```python
from build123d import *

# Parameters (mm, degrees)
F1_DEPTH = 15


with BuildPart() as f1:
    # F0 (on Front) → F1 (new body)
    with BuildSketch(Plane.XZ):
        with BuildLine():
            Line((177, 0), (0, 0))
            Line((0, 0), (0, -1337))
            Line((0, -1337), (274, -1337))
            Line((274, -1337), (274, -1212))
            ThreePointArc((274, -1212), (322.5253137442, -1088.8902928279), (442, -1032))
            Line((442, -1032), (442, -1000))
            Line((442, -1000), (480, -967))
            Line((480, -967), (480, -937))
            Line((480, -937), (477, -887))
            add(Edge.make_bspline(
                [(477, -887), (477.3409901345, -865.6929372181), (477.0797844675, -851.0610734518), (476.1022594588, -737.3138139423), (476.5777735361, -793.1899508202), (474.0967013355, -723.7578035301), (464.8329395432, -637.3258006514), (461.2628948716, -536.660924146), (443.9915396348, -436.9186876346), (426.5757756979, -336.5383755873), (399.3587210867, -237.3522036261), (375.4775408132, -133.8744354339), (355.455463807, -69.1251180104), (340, -27)],
                knots=[0, 0, 0, 0, 0.0728496243, 0.1620736999, 0.2013801511, 0.2662309643, 0.3694203367, 0.4725712376, 0.576170853, 0.6801132511, 0.7847115324, 0.8893098137, 1, 1, 1, 1], degree=3))
            Line((340, -27), (177, 0))
        make_face()
        with BuildLine():
            ThreePointArc((85, -582), (86.4644660941, -578.4644660941), (90, -577))
            Line((90, -577), (360, -577))
            ThreePointArc((360, -577), (363.5355339059, -578.4644660941), (365, -582))
            Line((365, -582), (365, -732))
            ThreePointArc((365, -732), (363.5355339059, -735.5355339059), (360, -737))
            Line((360, -737), (90, -737))
            ThreePointArc((90, -737), (86.4644660941, -735.5355339059), (85, -732))
            Line((85, -732), (85, -582))
        make_face(mode=Mode.SUBTRACT)
    extrude(amount=F1_DEPTH)


solid = f1.part
```
For this review, take the finished solid that the model builds, in its own axes (mm). Round coordinates to 2 decimals unless told otherwise and drop trailing zeros. Order: outer loops, then holes, each group sorted by start corner. A loop starts at its lowest first (then second) coordinate and runs counter-clockwise, first axis right, second up. Notation, with made-up numbers: (12, 64.5) -> (16, 64.5) arc R23 cw to (16, 84.5) -> close; hole circle Ø9 at (3, -4.75). An arc over 180 degrees is marked (long way). Use a Markdown table: item, result.
Item 1: For line 1 along Z through (x, y) = (99, -4.5); line 2 along Z through (x, y) = (324, -14); line 3 along X through (y, z) = (-9, -1021), list the stretches that pass through material, from the lowest coordinate up. Write a range as [from, to].
Resolved:
| item | result |
|---|---|
| line 1 | z = [-1337, -737], [-577, 0] |
| line 2 | z = [-1087.33, -737], [-577, -24.35] |
| line 3 | x = [0, 442] |
Item 2: For pin 1 (4 mm diameter, centred on x = 105.5, z = -1008.5, fed in from +Y); pin 2 (4 mm diameter, centred on y = -4, z = -525.5, fed in from +X); pin 3 (4 mm diameter, centred on x = 283, y = -3.5, fed in from +Z); pin 4 (5 mm diameter, centred on y = -6, z = -552, fed in from +X), all flat-tipped, find the tip position at first contact; note any pin that passes through.
Resolved:
| item | result |
|---|---|
| pin 1 | stops at y = 0 |
| pin 2 | stops at x = 457.95 |
| pin 3 | stops at z = -17.23 |
| pin 4 | stops at x = 460.62 |
Item 3: Take a section at A-A (x = 140.5). State the section outline as (y, z) points.
Resolved:
| item | result |
|---|---|
| outline | (-15, -1337) -> (0, -1337) -> (0, -737) -> (-15, -737) -> close; (-15, -577) -> (0, -577) -> (0, 0) -> (-15, 0) -> close |
Item 4: Take a section at B-B (x = 288). State the section outline as (y, z) points (1 decimal), plus the area to 3 significant figures.
Resolved:
| item | result |
|---|---|
| outline | (-15, -1142.3) -> (0, -1142.3) -> (0, -737) -> (-15, -737) -> close; (-15, -577) -> (0, -577) -> (0, -18.4) -> (-15, -18.4) -> close |
| area | 14,500 mm² |
